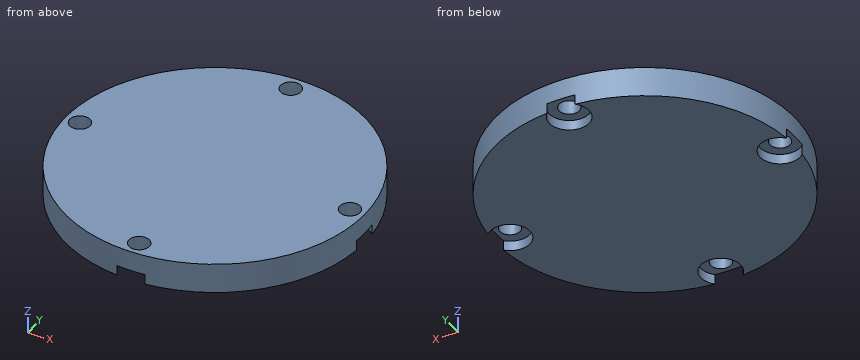
from build123d import *

# Parameters (mm, degrees)
SKETCH_1_R          = 15
EXTRUDE_1_DEPTH     = 3
SKETCH_2_R          = 1.025
CUT_EXTRUDE_2_DEPTH = 22.424285286
SKETCH_3_R          = 2
CUT_EXTRUDE_3_DEPTH = 1


with BuildPart() as part:
    # 草图1 → 凸台-拉伸1 (new body)
    with BuildSketch(Plane.XY):
        Circle(SKETCH_1_R)
    extrude(amount=EXTRUDE_1_DEPTH)

    # 草图2 → 切除-拉伸2 (cut, through all)
    with BuildSketch(Plane.XY):
        with Locations((0, 13.5)):
            Circle(SKETCH_2_R)
        with Locations((13.5, 0)):
            Circle(SKETCH_2_R)
        with Locations((0, -13.5)):
            Circle(SKETCH_2_R)
        with Locations((-13.5, 0)):
            Circle(SKETCH_2_R)
    extrude(amount=CUT_EXTRUDE_2_DEPTH, mode=Mode.SUBTRACT)

    # 草图3 → 切除-拉伸3 (cut)
    with BuildSketch(Plane(origin=(0, 0, 0), x_dir=(-1, 0, 0), z_dir=(0, 0, -1))):
        with Locations((0, 13.5)):
            Circle(SKETCH_3_R)
        with Locations((13.5, 0)):
            Circle(SKETCH_3_R)
        with Locations((-13.5, 0)):
            Circle(SKETCH_3_R)
        with Locations((0, -13.5)):
            Circle(SKETCH_3_R)
    extrude(amount=-CUT_EXTRUDE_3_DEPTH, mode=Mode.SUBTRACT)


solid = part.part
Can you work these out from the model? Positions are in its coordinate system, mm. Round coordinates to 2 decimals unless told otherwise and drop trailing zeros. Write each loop counter-clockwise with the first axis right and the second up, starting at its lowest first coordinate (ties: lowest second). Pieces come first, ordered by that corner, then holes. Notation, with made-up numbers: (48, -38) -> (55, -38) arc R11 ccw to (55, -20) -> close; hole circle Ø3 at (30.5, 83.25). An arc over 180 degrees is marked (long way). Use one line per item in the form item = value. Start each with the question number.
Q1. If I drill on probe 1 along X at (y, z) = (0, 1.9) (3 decimals); probe 2 along X at (y, z) = (-13.5, 1.95) (3 decimals), over which ranges is the centre line in solid material (lowest first)? Write a range as [from, to].
Q2. Imagine slicing it at D-D (y = -13.5). Please give me the cut outline in (x, z) (3 decimals), then the cut area to 3 significant figures.
Q3. Imagine slicing it at C-C (z = 2.5). Please give me the cut outline in (x, y) (3 decimals), then the cut area to 3 significant figures.
Q4. Imagine slicing it at A-A (x = 0). Please give me the cut outline in (y, z) (3 decimals).
Q5. I'm going to push flat-ended pins straight in: P1, Ø1.5, axis at y = -5.5, z = 1, coming from the +X side; P2, Ø1.5, axis at y = -1.5, z = 1.5, coming from the +X side. Where does each tip first touch, or does it pass through?
Worked out:
q1.probe_1 = [-15, -14.525], [-12.475, 12.475], [14.525, 15]
q1.probe_2 = [-6.538, -1.025], [1.025, 6.538]
q2.outline = (-6.538, 0) -> (-2, 0) -> (-2, 1) -> (-1.025, 1) -> (-1.025, 3) -> (-6.538, 3) -> close; (1.025, 1) -> (2, 1) -> (2, 0) -> (6.538, 0) -> (6.538, 3) -> (1.025, 3) -> close
q2.area = 31.1 mm^2
q3.outline = circle Ø30 at (0, 0); hole circle Ø2.05 at (-13.5, 0); hole circle Ø2.05 at (0, -13.5); hole circle Ø2.05 at (0, 13.5); hole circle Ø2.05 at (13.5, 0)
q3.area = 694 mm^2
q4.outline = (-15, 1) -> (-14.525, 1) -> (-14.525, 3) -> (-15, 3) -> close; (-12.475, 1) -> (-11.5, 1) -> (-11.5, 0) -> (11.5, 0) -> (11.5, 1) -> (12.475, 1) -> (12.475, 3) -> (-12.475, 3) -> close; (14.525, 1) -> (15, 1) -> (15, 3) -> (14.525, 3) -> close
q5.P1 = 14.23
q5.P2 = 14.98
